Design review of the part built by this model. Coordinates are the model's own, in mm. A direction names the side the tool comes from. Give positions to 0.01 mm unless a question says otherwise; leave off trailing zeros. Write each loop counter-clockwise with the first axis right and the second up, starting at its lowest first coordinate (ties: lowest second). Pieces come first, ordered by that corner, then holes. Notation, with made-up numbers: (-23, 85.25) -> (10, 85.25) arc R27 ccw to (10, 115.25) -> close; hole circle Ø7 at (-5.75, 15). An arc over 180 degrees is marked (long way). Use CSV: the item, a comma, the result in double quotes.
Autodesk Inventor part; units mm, degrees
ref_plane "YZ Plane" through (0, 0, 0) normal (1, 0, 0) x (0, 1, 0)
ref_plane "XZ Plane" through (0, 0, 0) normal (0, 1, 0) x (-1, 0, 0)
ref_plane "XY Plane" through (0, 0, 0) normal (0, 0, 1) x (1, 0, 0)
sketch "Sketch1" plane through (0, 0, 0) normal (0, 1, 0) x (-1, 0, 0)
  line L0 (0, 0) -> (50, 0)
  line L1 (50, 0) -> (50, 3)
  line L2 (0, 0) -> (0, 50)
  line L3 (0, 50) -> (3, 50)
  line L4 (3, 50) -> (3, 3)
  line L5 (3, 3) -> (50, 3)
  dimension "d0" = 50
  dimension "d1" = 3
  dimension "d2" = 50
  dimension "d3" = 3
extrude "Extrusion1" add sketch "Sketch1" along normal blind 660.4
sketch "Sketch2" plane through (-3, 0, 3) normal (-1, 0, 0) x (0, 0, 1)
  line L0 (0, 0) -> (47, 0)
  line L1 (-3, 0) -> (-3, 660.4)
  line L2 (-3, 13.8784) -> (9.7, 13.8784) construction
  line L3 (9.7, 0) -> (9.7, 15.7) construction
  line L4 (9.7, 0) -> (25.4, 0) construction
  line L5 (9.7, 15.7) -> (9.7, 91.9) construction
  line L6 (9.7, 91.9) -> (9.7, 168.1) construction
  line L7 (9.7, 168.1) -> (9.7, 244.3) construction
  line L8 (9.7, 244.3) -> (9.7, 320.5) construction
  line L9 (9.7, 320.5) -> (9.7, 396.7) construction
  line L10 (9.7, 396.7) -> (9.7, 472.9) construction
  line L11 (9.7, 472.9) -> (9.7, 549.1) construction
  line L12 (0, 660.4) -> (47, 660.4) construction
  line L13 (9.7, 661.3513) -> (9.7, 645.6513) construction
  line L14 (9.7, 549.1) -> (9.7, 625.3) construction
  circle A0 centre (9.7, 645.6513) radius 3.175
  circle A1 centre (9.7, 549.1) radius 3.175
  circle A2 centre (9.7, 472.9) radius 3.175
  circle A3 centre (9.7, 396.7) radius 3.175
  circle A4 centre (9.7, 320.5) radius 3.175
  circle A5 centre (9.7, 244.3) radius 3.175
  circle A6 centre (9.7, 168.1) radius 3.175
  circle A7 centre (9.7, 91.9) radius 3.175
  circle A8 centre (9.7, 13.8784) radius 3.175
  dimension "d26" = 12.7
  dimension "d28" = 15.7
  dimension "d29" = 90
  dimension "d30" = 76.2
  dimension "d31" = 180
  dimension "d32" = 76.2
  dimension "d33" = 180
  dimension "d34" = 76.2
  dimension "d35" = 180
  dimension "d36" = 76.2
  dimension "d37" = 180
  dimension "d38" = 76.2
  dimension "d39" = 180
  dimension "d40" = 76.2
  dimension "d41" = 180
  dimension "d42" = 76.2
  dimension "d43" = 180
  dimension "d44" = 15.7
  dimension "d45" = 76.2
  dimension "d46" = 6.35
  dimension "d47" = 6.35
  dimension "d48" = 6.35
  dimension "d49" = 6.35
  dimension "d50" = 6.35
  dimension "d51" = 6.35
  dimension "d52" = 6.35
  dimension "d53" = 6.35
  dimension "d54" = 6.35
extrude "Extrusion2" cut sketch "Sketch2" against normal blind 25.4
properties part number "26in Angle Channel" material "Aluminum 6061"
(1) Take a section at B-B (x = -28.5). Write out the cut boundary in (y, z), then the cut area to 3 significant figures.
Established:
outline,"(0, 0) -> (660.4, 0) -> (660.4, 3) -> (0, 3) -> close"
area,"1,980 mm2"
(2) Tool access review of faces 1 (the face through (-3, 326, 27)), 2 (the face through (-2.7, 660.4, 14)): name each direction out of +Z, -Z, +X, -X, +Y, -Y from which nothing blocks a thin tool from reaching the whole face with its end or side.
Established:
face 1,"+Z, -X, +Y, -Y"
face 2,"+Z, -Z, +X, -X, +Y"
(3) Clearance check with flat-ended pins moving along their axes: pin 1 (5.5 mm diameter, centred on y = 320.5, z = 12.7, fed in from -X); pin 2 (1.5 mm diameter, centred on y = 148, z = 22.5, fed in from -X); pin 3 (10 mm diameter, centred on x = -30.5, y = 335.5, fed in from +Z). State where each tip first meets the part, or that it passes through.
Established:
pin 1,"passes through"
pin 2,"stops at x = -3"
pin 3,"stops at z = 3"
(4) Take a section at C-C (z = 32.5). Write out the cut boundary in (x, y).
Established:
outline,"(-3, 0) -> (0, 0) -> (0, 660.4) -> (-3, 660.4) -> close"
(5) For line 1 along Z through (x, y) = (-0.6, 168.1) (3 decimals); line 2 along X through (y, z) = (69, 20.5); line 3 along Z through (x, y) = (-23, 451), list the stretches that pass through material, from the lowest coordinate up. Write a range as [from, to].
Established:
line 1,"z = [0, 9.525], [15.875, 50]"
line 2,"x = [-3, 0]"
line 3,"z = [0, 3]"
(6) Take a section at A-A (y = 387). Write out the cut boundary in (x, z), then the cut area to 3 significant figures.
Established:
outline,"(-50, 0) -> (0, 0) -> (0, 50) -> (-3, 50) -> (-3, 3) -> (-50, 3) -> close"
area,"291 mm2"
